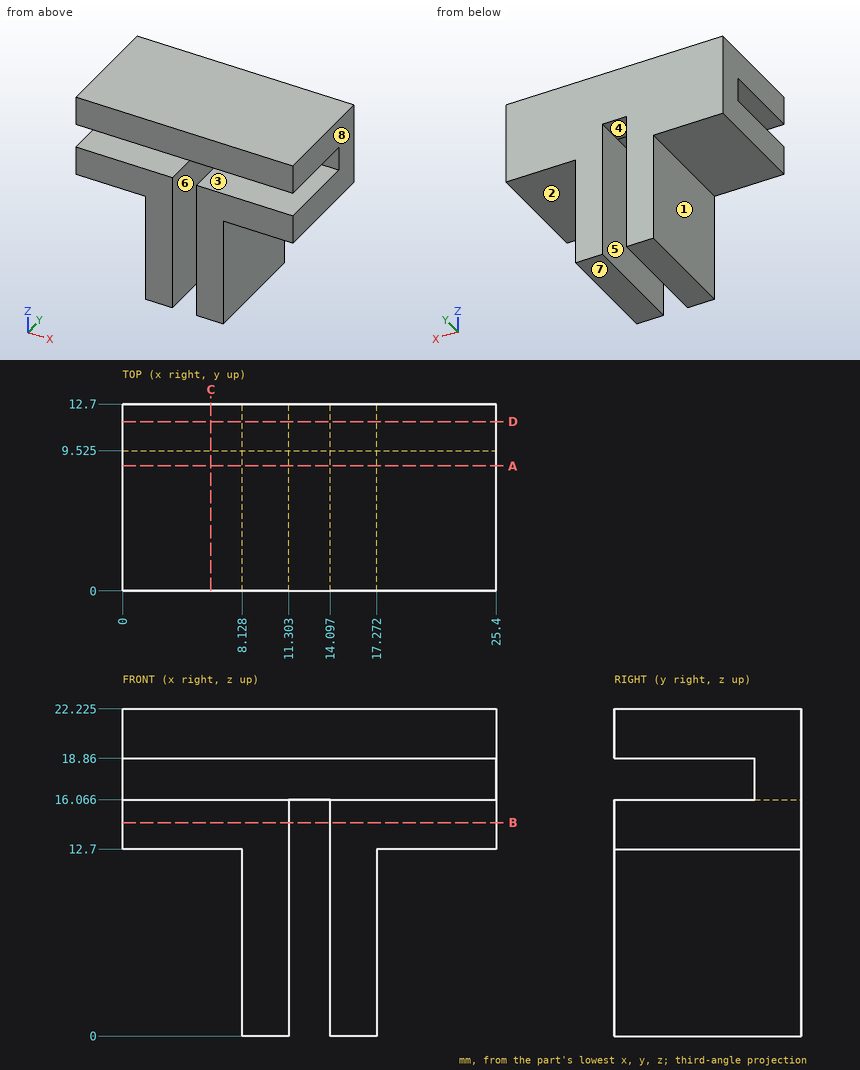
The drawing under review shows one solid part. Ordinate dimensions are in mm from its lowest x, y, z. A direction names the side the tool comes from. Round coordinates to 2 decimals unless told otherwise and drop trailing zeros. Loops run counter-clockwise (first coordinate to the right, second up) from the corner with the lowest first, then second, coordinate; pieces in that order, holes last. Notation, with made-up numbers: (-32.75, 12.25) - (-25.75, 12.25) arc R9 cw to (-25.75, 21.25) - close; hole circle Ø9 at (-31.75, -36). An arc over 180 degrees is marked (long way). Put each result on its own line as item: value. Start each with the question number.
1. Mouldability with a two-part tool opening along X and no side actions: class the marked faces 5, 6, 7 and 8 as +X half, -X half, draft (parallel to the pull), parting line (faces both ways), or undercut.
2. Consider section C-C on x = 6. State the section outline as (y, z) points (1 decimal).
3. Consider section D-D on y = 11.5. State the section outline as (x, z) points (1 decimal).
4. Consider section A-A on y = 8.5. State the section outline as (x, z) points (1 decimal).
5. For probe 1 along Z at (x, y) = (20.25, 4.5) (1 decimal); probe 2 along X at (y, z) = (10.75, 3.25); probe 3 along Z at (x, y) = (10.5, 2) (1 decimal), list the stretches that pass through material, from the lowest coordinate up. Write a range as [from, to].
6. Consider section B-B on z = 14.5. State the section outline as (x, y) points.
7. Insertion check: P1, Ø0.8, axis at x = 10, z = 18, coming from the -Y side (1 decimal); P2, Ø4, axis at x = 2, y = 8.5, coming from the -Z side. Each pin has a flat end and moves straight along its axis. Give the tip position at first contact, or say it passes through.
8. For the marked faces 1, 2, 3 and 4, list the 3-axis set-ups (+Z, -Z, +X, -X, +Y, -Y) from which the entire face can be reached by the end or side of a thin tool; tool diameter is ignored.
Result sheet:
1. face 5: undercut
1. face 6: undercut
1. face 7: draft
1. face 8: +X half
2. outline: (0, 12.7) - (12.7, 12.7) - (12.7, 22.2) - (0, 22.2) - (0, 18.9) - (9.5, 18.9) - (9.5, 16.1) - (0, 16.1) - close
3. outline: (0, 12.7) - (8.1, 12.7) - (8.1, 0) - (11.3, 0) - (11.3, 16.1) - (14.1, 16.1) - (14.1, 0) - (17.3, 0) - (17.3, 12.7) - (25.4, 12.7) - (25.4, 22.2) - (0, 22.2) - close
4. outline: (0, 12.7) - (8.1, 12.7) - (8.1, 0) - (11.3, 0) - (11.3, 16.1) - (0, 16.1) - close; (0, 18.9) - (25.4, 18.9) - (25.4, 22.2) - (0, 22.2) - close; (14.1, 0) - (17.3, 0) - (17.3, 12.7) - (25.4, 12.7) - (25.4, 16.1) - (14.1, 16.1) - close
5. probe 1: [12.7, 16.1], [18.9, 22.2]
5. probe 2: [8.13, 11.3], [14.1, 17.27]
5. probe 3: [0, 16.1], [18.9, 22.2]
6. outline: (0, 0) - (11.3, 0) - (11.3, 12.7) - (0, 12.7) - close; (14.1, 0) - (25.4, 0) - (25.4, 12.7) - (14.1, 12.7) - close
7. P1: y = 9.5
7. P2: z = 12.7
8. face 1: -Z, -X, +Y, -Y
8. face 2: -Z, +X, +Y, -Y
8. face 3: +X, -X, -Y
8. face 4: -Z, +Y, -Y
